from build123d import *

# Parameters (mm, degrees)
BOSS_EXTRUDE1_DEPTH = 50
SKETCH2_R           = 20
BOSS_EXTRUDE2_DEPTH = 20
BOSS_EXTRUDE3_START = 20
SKETCH3_R           = 20
BOSS_EXTRUDE3_DEPTH = 20
SKETCH4_R           = 20
CUT_EXTRUDE1_DEPTH  = 70
SKETCH5_R           = 20
CUT_EXTRUDE2_DEPTH  = 70
FILLET1_R           = 10


with BuildPart() as part:
    # Sketch1 → Boss-Extrude1 (new body)
    with BuildSketch(Plane.XY):
        Polygon((-76.447024941, -6.493075274), (-76.447024941, 87.506924726), (58.552975059, 87.506924726), (58.552975059, 307.506924726), (118.552975059, 307.506924726), (118.552975059, 87.506924726), (618.552975059, 87.506924726), (618.552975059, 307.506924726), (678.552975059, 307.506924726), (678.552975059, 87.506924726), (1373.552975059, 87.506924726), (1373.552975059, -6.493075274), align=None)
    extrude(amount=BOSS_EXTRUDE1_DEPTH)

    # Sketch2 → Boss-Extrude2 (add)
    with BuildSketch(Plane.ZY.offset(76.447024941)):
        with Locations((25, 40.506924726)):
            Circle(SKETCH2_R)
    extrude(amount=BOSS_EXTRUDE2_DEPTH)

    # Sketch3 → Boss-Extrude3 (add)
    with BuildSketch(Plane(origin=(1373.552975059, 0, 0), x_dir=(0, 0, -1), z_dir=(1, 0, 0)).offset(BOSS_EXTRUDE3_START)):
        with Locations(Location((-25, 40.506924726, 0), (0, 0, 180))):
            Circle(SKETCH3_R)
    extrude(amount=-BOSS_EXTRUDE3_DEPTH)

    # Sketch4 → Cut-Extrude1 (cut)
    with BuildSketch(Plane.XY.offset(50)):
        with Locations((88.552975059, 282.506924726)):
            Circle(SKETCH4_R)
    extrude(amount=-CUT_EXTRUDE1_DEPTH, mode=Mode.SUBTRACT)

    # Sketch5 → Cut-Extrude2 (cut)
    with BuildSketch(Plane.XY.offset(50)):
        with Locations((648.552975059, 282.506924726)):
            Circle(SKETCH5_R)
    extrude(amount=-CUT_EXTRUDE2_DEPTH, mode=Mode.SUBTRACT)

    # Fillet1
    # the kernel refuses this fillet: 10 mm, written as the material it takes off along each edge
    with BuildSketch(Plane(origin=(33.552975059, 307.506924726, 0), x_dir=(0, -1, 0), z_dir=(1, 0, 0)), Plane(origin=(593.552975059, 307.506924726, 0), x_dir=(0, -1, 0), z_dir=(1, 0, 0))) as fillet1_piece_1:
        with BuildLine():
            CenterArc((FILLET1_R, -FILLET1_R), FILLET1_R, 90, 90)
            Line((0, -FILLET1_R), (0, 0))
            Line((0, 0), (FILLET1_R, 0))
        make_face()
    extrude(amount=110, mode=Mode.SUBTRACT)
    with BuildSketch(Plane(origin=(593.552975059, 307.506924726, 50), x_dir=(0, -1, 0), z_dir=(1, 0, 0)), Plane(origin=(33.552975059, 307.506924726, 50), x_dir=(0, -1, 0), z_dir=(1, 0, 0))) as fillet1_piece_2:
        with BuildLine():
            CenterArc((FILLET1_R, FILLET1_R), FILLET1_R, 180, 90)
            Line((0, FILLET1_R), (0, 0))
            Line((0, 0), (FILLET1_R, 0))
        make_face()
    extrude(amount=110, mode=Mode.SUBTRACT)
    with BuildSketch(Plane(origin=(58.552975059, 307.506924726, -25), x_dir=(0, -1, 0), z_dir=(0, 0, 1)), Plane(origin=(118.552975059, 307.506924726, -25), x_dir=(-1, 0, 0), z_dir=(0, 0, 1))) as fillet1_piece_3:
        with BuildLine():
            CenterArc((FILLET1_R, FILLET1_R), FILLET1_R, 180, 90)
            Line((0, FILLET1_R), (0, 0))
            Line((0, 0), (FILLET1_R, 0))
        make_face()
    extrude(amount=100, mode=Mode.SUBTRACT)
    with BuildSketch(Plane(origin=(618.552975059, 307.506924726, -25), x_dir=(1, 0, 0), z_dir=(0, 0, 1)), Plane(origin=(678.552975059, 307.506924726, -25), x_dir=(0, -1, 0), z_dir=(0, 0, 1))) as fillet1_piece_4:
        with BuildLine():
            CenterArc((FILLET1_R, -FILLET1_R), FILLET1_R, 90, 90)
            Line((0, -FILLET1_R), (0, 0))
            Line((0, 0), (FILLET1_R, 0))
        make_face()
    extrude(amount=100, mode=Mode.SUBTRACT)


solid = part.part
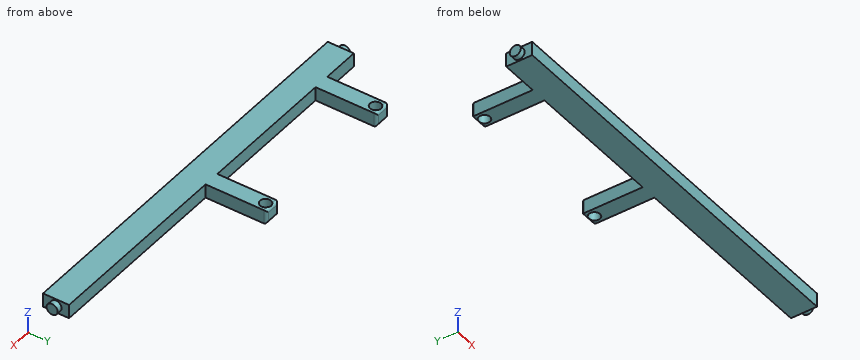
The model under review builds one solid part; all positions refer to its coordinate system, in mm. Round coordinates to 2 decimals unless told otherwise and drop trailing zeros. Order: outer loops, then holes, each group sorted by start corner. A loop starts at its lowest first (then second) coordinate and runs counter-clockwise, first axis right, second up. Notation, with made-up numbers: (56.25, 18) - (70.25, 18) arc R28 ccw to (70.25, 37) - close; hole circle Ø7 at (-36, 9). An arc over 180 degrees is marked (long way). Use one line per item in the form item = value.
Q1. Add section C-C on x = 577. Give the boundary of the cut face in (y, z), then the cut area to 3 significant figures.
Response values:
outline = (-6.49, 0) - (87.51, 0) - (87.51, 50) - (-6.49, 50) - close
area = 4,700 mm^2
Q2. To check wall thickness, follow line 1 (X direction, y = 229.5, z = 10); line 2 (X direction, y = 265, z = 17); line 3 (X direction, y = 84, z = 38.5). State the ranges of each line that lie inside material, in increasing order.
Response values:
line_1 = 58.55 to 118.55, 618.55 to 678.55
line_2 = 58.55 to 78.88, 98.22 to 118.55, 618.55 to 638.88, 658.22 to 678.55
line_3 = -76.45 to 1373.55
Q3. Clearance check with flat-ended pins moving along their axes: P1, Ø15, axis at y = 149.5, z = 22, coming from the -X side; P2, Ø12, axis at y = 210.5, z = 34, coming from the +X side; P3, Ø15, axis at x = 1169.5, z = 16, coming from the +Y side; P4, Ø25, axis at y = 20.5, z = 28, coming from the +X side. State where each tip first meets the part, or that it passes through.
Response values:
P1 = 58.55
P2 = 678.55
P3 = 87.51
P4 = 1393.55
Q4. Add section A-A on y = 236. Give the boundary of the cut face in (x, z).
Response values:
outline = (58.55, 0) - (118.55, 0) - (118.55, 50) - (58.55, 50) - close; (618.55, 0) - (678.55, 0) - (678.55, 50) - (618.55, 50) - close
Q5. Add section B-B on z = 27.5. Give the boundary of the cut face in (x, y), then the cut area to 3 significant figures.
Response values:
outline = (-96.45, 20.66) - (-76.45, 20.66) - (-76.45, -6.49) - (1373.55, -6.49) - (1373.55, 20.66) - (1393.55, 20.66) - (1393.55, 60.35) - (1373.55, 60.35) - (1373.55, 87.51) - (678.55, 87.51) - (678.55, 297.51) arc R10 ccw to (668.55, 307.51) - (628.55, 307.51) arc R10 ccw to (618.55, 297.51) - (618.55, 87.51) - (118.55, 87.51) - (118.55, 297.51) arc R10 ccw to (108.55, 307.51) - (68.55, 307.51) arc R10 ccw to (58.55, 297.51) - (58.55, 87.51) - (-76.45, 87.51) - (-76.45, 60.35) - (-96.45, 60.35) - close; hole circle Ø40 at (88.55, 282.51); hole circle Ø40 at (648.55, 282.51)
area = 162,000 mm^2
